```python
from build123d import *

# Parameters (mm, degrees)
BASE_EXTRUDE_DEPTH = 12.7
CIRPATTERN1_COUNT  = 2


with BuildPart() as part:
    # Sketch1 → Base-Extrude (new, symmetric)
    with BuildSketch(Plane.XY):
        with BuildLine():
            Line((-41.275, 15.875), (-41.275, -17.9451))
            ThreePointArc((-41.275, -17.9451), (-40.486414298, -19.848914298), (-38.5826, -20.6375))
            Line((-38.5826, -20.6375), (-2.6924, -20.6375))
            ThreePointArc((-2.6924, -20.6375), (-0.788585702, -19.848914298), (0, -17.9451))
            Line((0, -17.9451), (0, 15.875))
            ThreePointArc((0, 15.875), (-4.7625, 20.6375), (-9.525, 15.875))
            Line((-9.525, 15.875), (-9.525, 14.83995))
            ThreePointArc((-9.525, 14.83995), (-8.1788, 13.49375), (-6.8326, 14.83995))
            Line((-6.8326, 14.83995), (-6.8326, 15.875))
            ThreePointArc((-6.8326, 15.875), (-4.7625, 17.9451), (-2.6924, 15.875))
            Line((-2.6924, 15.875), (-2.6924, -17.9451))
            Line((-2.6924, -17.9451), (-38.5826, -17.9451))
            Line((-38.5826, -17.9451), (-38.5826, 15.875))
            ThreePointArc((-38.5826, 15.875), (-36.5125, 17.9451), (-34.4424, 15.875))
            Line((-34.4424, 15.875), (-34.4424, 14.83995))
            ThreePointArc((-34.4424, 14.83995), (-33.0962, 13.49375), (-31.75, 14.83995))
            Line((-31.75, 14.83995), (-31.75, 15.875))
            ThreePointArc((-31.75, 15.875), (-36.5125, 20.6375), (-41.275, 15.875))
        make_face()
    base_extrude = extrude(amount=BASE_EXTRUDE_DEPTH, both=True)

    # CirPattern1: Base-Extrude ×2 about axis
    cirpattern1_axis = Axis((0, 0, 0), (0, 0, 1))
    for i in range(1, CIRPATTERN1_COUNT):
        add(base_extrude.rotate(cirpattern1_axis, i * 360 / CIRPATTERN1_COUNT))


solid = part.part
```
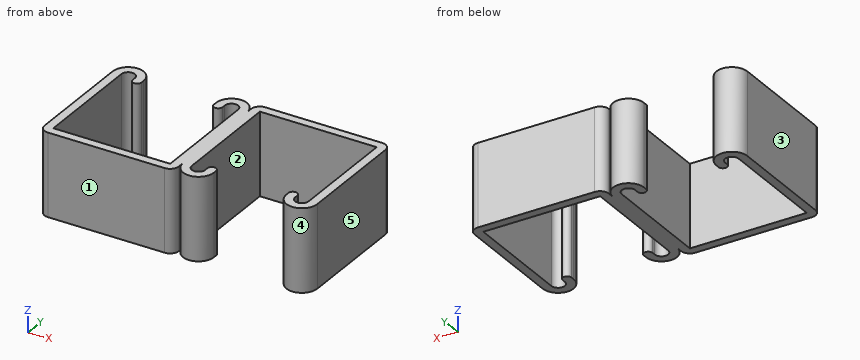
Work out the finished part from the listing and answer in its coordinate system (mm). Face numbers are marked on the shaded views. A direction names the side the tool comes from. Coordinates: 2 decimals unless noted, no trailing zeros. Loops run counter-clockwise (first coordinate to the right, second up) from the corner with the lowest first, then second, coordinate; pieces in that order, holes last. Notation, with made-up numbers: M -28,1.5 L 19,1.5 A26 cw 19,37.5 Z; hole C -33.75,-19 d6. An arc over 180 degrees is marked long. Use CSV: the item, a comma, the result in double quotes. Start each with the question number.
(1) Consider line 1 (X direction, y = 12.5, z = 5.5) (3 decimals); line 2 (X direction, y = -15, z = 7.5) (3 decimals); line 3 (Y direction, x = -36.5, z = 0). Determine where each line is inside the solid, lowest interval first.
(2) Given pin 1 Ø5 at (x, y) = (17.5, 14.5) entering from +Z; pin 2 Ø0.6 at (y, z) = (-17, -1.5) entering from +X; pin 3 Ø0.6 at (y, z) = (17.5, -1) entering from -X, each flat-ended and moving along its own axis, determine where each tip first touches the part or whether it passes through.
(3) Find section B-B, the plane y = -17. Give the vertices of the cut face in (x, z) (3 decimals).
(4) Find section C-C, the plane x = 13.5. Give the vertices of the cut face in (y, z), then the cut area to 3 significant figures.
(5) For a pull along X with two mould halves and no side action, classify the marked faces 3, 4 and 5 as +X half, -X half, draft (parallel to the pull), parting line (faces both ways), or undercut.
(6) For the marked faces 1 and 2, determine the directions among +Z, -Z, +X, -X, +Y, -Y from which every point of the face is accessible in a straight line to the end or side of a thin tool.
(7) Find section A-A, the plane y = -3. Give the vertices of the cut face in (x, z) (3 decimals), then the cut area to 3 significant figures.
Recorded:
1,line 1,"x = -41.275 to -38.583, -2.692 to 2.692, 38.583 to 41.275"
1,line 2,"x = -41.275 to -38.583, -2.692 to 2.692, 6.833 to 9.525, 31.75 to 34.442, 38.583 to 41.275"
1,line 3,"y = -20.64 to -17.95, 17.95 to 20.64"
2,pin 1,"passes through"
2,pin 2,"stops at x = 41.2"
2,pin 3,"stops at x = -41.09"
3,outline,"M -41.275,-12.7 L -38.583,-12.7 L -38.583,12.7 L -41.275,12.7 Z; M -2.692,-12.7 L 0,-12.7 L 0,12.7 L -2.692,12.7 Z; M 0.135,-12.7 L 3.025,-12.7 L 3.025,12.7 L 0.135,12.7 Z; M 6.5,-12.7 L 9.39,-12.7 L 9.39,12.7 L 6.5,12.7 Z; M 31.885,-12.7 L 34.775,-12.7 L 34.775,12.7 L 31.885,12.7 Z; M 38.25,-12.7 L 41.14,-12.7 L 41.14,12.7 L 38.25,12.7 Z"
4,outline,"M 17.95,-12.7 L 20.64,-12.7 L 20.64,12.7 L 17.95,12.7 Z"
4,area,"68.4 mm^2"
5,face 3,"-X half"
5,face 4,"undercut"
5,face 5,"+X half"
6,face 1,"+Z, -Z, +X, -X, -Y"
6,face 2,"+Z, -Z"
7,outline,"M -41.275,-12.7 L -38.583,-12.7 L -38.583,12.7 L -41.275,12.7 Z; M -2.692,-12.7 L 2.692,-12.7 L 2.692,12.7 L -2.692,12.7 Z; M 38.583,-12.7 L 41.275,-12.7 L 41.275,12.7 L 38.583,12.7 Z"
7,area,"274 mm^2"
